Can you work these out from the model? Positions are in its coordinate system, mm. Face numbers are marked on the shaded views. A direction names the side the tool comes from. Round coordinates to 2 decimals unless told otherwise and drop trailing zeros. Order: outer loops, then holes, each group sorted by start corner. A loop starts at its lowest first (then second) coordinate and runs counter-clockwise, first axis right, second up. Notation, with made-up numbers: (86, 62.25) -> (130, 62.25) arc R27 ccw to (130, 81.25) -> close; hole circle Ø6 at (22, 87). An arc over 180 degrees is marked (long way). Use a Markdown table: item, result. Add a question column.
Q1. If we section it at A-A on y = 7.25: List the corners of the cut face in (x, z) for me.
Q2. If we section it at C-C on y = 5: List the corners of the cut face in (x, z) for me.
Q3. I need wall thicknesses on line 1 along Z through (x, y) = (6, 7); line 2 along Z through (x, y) = (6, 6.1); line 3 along X through (y, z) = (6, -46.5). Which ranges of each line are inside material? Lowest first, please. Write a range as [from, to].
Q4. If we section it at D-D on z = -48: List the corners of the cut face in (x, y) for me.
Q5. If we section it at B-B on x = 6: List the corners of the cut face in (y, z) for me, plus the area to 3 significant figures.
Q6. For the marked faces 1, 2 and 3, which set-ups out of +Z, -Z, +X, -X, +Y, -Y let a thin tool reach every point of the face, with its end or its side?
Q7. We'd pull the mould along X, two halves only. Please class the marked faces 4, 5 and 6: +X half, -X half, draft (parallel to the pull), parting line (faces both ways), or undercut.
Q8. I'm going to push flat-ended pins straight in: pin 1 Ø2.5 at (x, z) = (6, -46.5) entering from +Y; pin 2 Ø1.6 at (x, z) = (6, -46.5) entering from +Y; pin 3 Ø5.5 at (x, z) = (1.5, -24.5) entering from +Y; pin 4 Ø1.5 at (y, z) = (8, -48.5) entering from -X. Where does each tip first touch, or does it pass through?
```python
from build123d import *

# Parameters (mm, degrees)
SKETCH1_R           = 1
BOSS_EXTRUDE1_DEPTH = 8
SKETCH2_R           = 7
SKETCH2_R_2         = 3
CUT_EXTRUDE1_DEPTH  = 4
SKETCH3_R           = 3
CUT_EXTRUDE2_DEPTH  = 1.5
CUT_EXTRUDE3_DEPTH  = 4
BOSS_EXTRUDE2_START = -10
SKETCH5_W           = 30
SKETCH5_H           = 2
BOSS_EXTRUDE2_DEPTH = 2
SKETCH6_R           = 3
SKETCH6_R_2         = 1
BOSS_EXTRUDE3_DEPTH = 6
SKETCH7_R           = 1
CUT_EXTRUDE4_DEPTH  = 5


with BuildPart() as part:
    # Sketch1 → Boss-Extrude1 (new body)
    with BuildSketch(Plane(origin=(0, 0, 0), x_dir=(1, 0, 0), z_dir=(0, 1, 0))):
        with BuildLine():
            Line((-3, 53.504881109), (15, 53.504881109))
            Line((15, 53.504881109), (15, 23.504881109))
            ThreePointArc((15, 23.504881109), (6, 14.504881109), (-3, 23.504881109))
            Line((-3, 23.504881109), (-3, 53.504881109))
        make_face()
        with Locations((6, 36.504881109)):
            Circle(SKETCH1_R, mode=Mode.SUBTRACT)
        with Locations((6, 46.504881109)):
            Circle(SKETCH1_R, mode=Mode.SUBTRACT)
    extrude(amount=BOSS_EXTRUDE1_DEPTH)

    # Sketch2 → Cut-Extrude1 (cut)
    with BuildSketch(Plane(origin=(0, 8, 0), x_dir=(1, 0, 0), z_dir=(0, 1, 0))):
        with Locations((6, 23.504881109)):
            Circle(SKETCH2_R)
        with Locations((6, 23.504881109)):
            Circle(SKETCH2_R_2, mode=Mode.SUBTRACT)
    extrude(amount=-CUT_EXTRUDE1_DEPTH, mode=Mode.SUBTRACT)

    # Sketch3 → Cut-Extrude2 (cut)
    with BuildSketch(Plane(origin=(0, 8, 0), x_dir=(1, 0, 0), z_dir=(0, 1, 0))):
        with Locations((6, 23.504881109)):
            Circle(SKETCH3_R)
    extrude(amount=-CUT_EXTRUDE2_DEPTH, mode=Mode.SUBTRACT)

    # Sketch4 → Cut-Extrude3 (cut)
    with BuildSketch(Plane(origin=(0, 8, 0), x_dir=(1, 0, 0), z_dir=(0, 1, 0))):
        with BuildLine():
            Line((-4, 46.504881109), (-4, 53.993644797))
            Line((-4, 53.993644797), (16, 53.993644797))
            Line((16, 53.993644797), (16, 46.504881109))
            ThreePointArc((16, 46.504881109), (6, 36.504881109), (-4, 46.504881109))
        make_face()
    extrude(amount=-CUT_EXTRUDE3_DEPTH, mode=Mode.SUBTRACT)

    # Sketch5 → Boss-Extrude2 (add)
    with BuildSketch(Plane(origin=(15, 0, 0), x_dir=(0, 0, -1), z_dir=(1, 0, 0)).offset(BOSS_EXTRUDE2_START)):
        with Locations((38.504881109, 1)):
            Rectangle(SKETCH5_W, SKETCH5_H)
    extrude(amount=BOSS_EXTRUDE2_DEPTH)

    # Sketch6 → Boss-Extrude3 (add)
    with BuildSketch(Plane(origin=(0, 4, 0), x_dir=(1, 0, 0), z_dir=(0, 1, 0))):
        with Locations((6, 46.504881109)):
            Circle(SKETCH6_R)
        with Locations((6, 46.504881109)):
            Circle(SKETCH6_R_2, mode=Mode.SUBTRACT)
    extrude(amount=BOSS_EXTRUDE3_DEPTH)

    # Sketch7 → Cut-Extrude4 (cut)
    with BuildSketch(Plane(origin=(0, 0, -53.504881109), x_dir=(-1, 0, 0), z_dir=(0, 0, -1))):
        with Locations((-12, 2)):
            Circle(SKETCH7_R)
        with Locations((0, 2)):
            Circle(SKETCH7_R)
    extrude(amount=-CUT_EXTRUDE4_DEPTH, mode=Mode.SUBTRACT)


solid = part.part
```
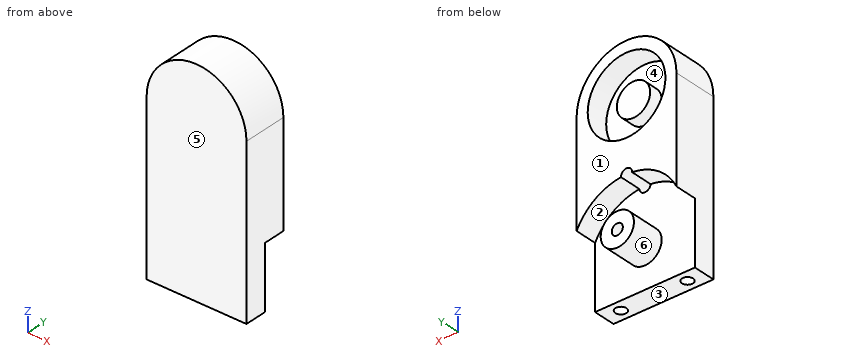
Answer below:
| question | item | result |
|---|---|---|
| 1 | outline | (-3, -42.15) arc R10 cw to (5, -36.55) arc R1 cw (long way) to (7, -36.55) arc R10 cw to (15, -42.15) -> (15, -23.5) arc R9 ccw to (-3, -23.5) -> close; circle Ø6 at (6, -46.5); hole circle Ø14 at (6, -23.5); hole circle Ø2 at (6, -46.5) |
| 2 | outline | (-3, -42.15) arc R10 cw to (5, -36.55) arc R1 cw (long way) to (7, -36.55) arc R10 cw to (15, -42.15) -> (15, -23.5) arc R9 ccw to (-3, -23.5) -> close; circle Ø6 at (6, -46.5); circle Ø6 at (6, -23.5); hole circle Ø14 at (6, -23.5); hole circle Ø2 at (6, -46.5) |
| 3 | line 1 | [-49.5, -47.5], [-45.5, -43.5], [-35.5, -30.5], [-16.5, -14.5] |
| 3 | line 2 | [-49.5, -47.5], [-45.5, -43.5], [-35.5, -30.5], [-26.5, -20.5], [-16.5, -14.5] |
| 3 | line 3 | [3, 5], [7, 9] |
| 4 | outline | (-3, 0) -> (15, 0) -> (15, 4) -> (8.6, 4) -> (8.6, 10) -> (3.4, 10) -> (3.4, 4) -> (-3, 4) -> close |
| 5 | outline | (0, -53.5) -> (4, -53.5) -> (4, -49.5) -> (10, -49.5) -> (10, -47.5) -> (2, -47.5) -> (2, -45.5) -> (10, -45.5) -> (10, -43.5) -> (4, -43.5) -> (4, -37.5) -> (2, -37.5) -> (2, -35.5) -> (8, -35.5) -> (8, -30.5) -> (4, -30.5) -> (4, -26.5) -> (6.5, -26.5) -> (6.5, -20.5) -> (4, -20.5) -> (4, -16.5) -> (8, -16.5) -> (8, -14.5) -> (0, -14.5) -> close |
| 5 | area | 215 mm² |
| 6 | face 1 | +Z, +X, -X, +Y |
| 6 | face 2 | +Y |
| 6 | face 3 | -Z, +X, -X, +Y, -Y |
| 7 | face 4 | undercut |
| 7 | face 5 | draft |
| 7 | face 6 | parting line |
| 8 | pin 1 | y = 10 |
| 8 | pin 2 | y = 2 |
| 8 | pin 3 | y = 8 |
| 8 | pin 4 | x = 3.27 |
